Model file for the job. Use its own axes, mm. A direction names the side the tool comes from. Coordinates: 2 decimals unless noted, no trailing zeros. Order: outer loops, then holes, each group sorted by start corner. A loop starts at its lowest first (then second) coordinate and runs counter-clockwise, first axis right, second up. Notation, with made-up numbers: (88, 45) -> (115, 45) arc R24 cw to (115, 76) -> close; hole circle Ø5 at (17, 63.5). An arc over 180 degrees is marked (long way). Use CSV: the item, a comma, the result in double quotes. Start each with the question number.
(1) Cut at D-D on x = 20.5. Write the cut outline in (y, z), plus the area to 3 significant figures.
(2) Cut at B-B on x = 30.5. Write the cut outline in (y, z).
(3) Tool access for faces 4 (the flat face through (-12, -19, 3)), 5 (the cylindrical face through (-19.22, -24.79, 18.5)), 6 (the flat face through (-28, -20, 7.297)): list every direction of +Z, -Z, +X, -X, +Y, -Y with a clear straight run to the whole face (end or side of a thin tool).
(4) Probe L1, parallel to X at y = -21.5, z = 15; L2, parallel to X at y = -25.55, z = 17; L3, parallel to Y at x = 41, z = 17.25. List the from-to ranges inside material, lowest first.
(5) Cut at C-C on z = 10.25. Give the number of separate pieces and of enclosed holes in the cut face, plus the area to 3 significant figures.
(6) Pull direction Z, two halves, no side cores. Call faces 1 (the flat face through (-31, -16, 17)), 2 (the flat face through (-31, -28, 12)), 3 (the conical face through (40.656, 18.045, 6.007)): pulls with the +Z half, pulls with the -Z half, needs draft (parallel to the pull), parting line crosses it, or undercut.
(7) Pin check, flat tips, straight feed: pin 1 Ø4 at (x, z) = (15, 4) entering from -Y; pin 2 Ø1 at (x, y) = (12.5, -26) entering from +Z; pin 3 Ø3 at (x, z) = (-34.5, 14) entering from -Y; pin 4 Ø1.5 at (x, y) = (24.5, -17) entering from -Z. Stop position of each tip, or through.
(8) Cut at A-A on y = -20. Write the cut outline in (x, z), plus the area to 3 significant figures.
```python
from build123d import *

# Parameters (mm, degrees)
SKETCH1_W            = 92
SKETCH1_H            = 55
BODY_DEPTH           = 25
SKETCH2_R            = 9.75
BATTERY_DEPTH        = 37
SKETCH3_W            = 33
SKETCH3_H            = 8
CONTROLLER_DEPTH     = 22
CUT_EXTRUDE3_REACH   = 77.934
SKETCH4_R            = 4
CONNECTOR_REACH      = 77.934
SKETCH5_W            = 9
SKETCH5_H            = 10.5
SKETCH6_W            = 26
SKETCH6_H            = 6
CHARGER_DEPTH        = 22
CHGLED_REACH         = 77.934
SKETCH7_R            = 1.5
SKETCH8_W            = 20
SKETCH8_H            = 25
BOSS_EXTRUDE1_DEPTH  = 6
BOSS_EXTRUDE1_TAPER  = 30
SKETCH9_W            = 10
SKETCH9_H            = 14
CUT_EXTRUDE7_DEPTH   = 15
SKETCH10_W           = 8.515500197
SKETCH10_H           = 4.030526349
CUT_EXTRUDE8_DEPTH   = 15
SKETCH11_W           = 3
SKETCH11_H           = 48.5
CUT_EXTRUDE9_DEPTH   = 102.050729983
LPATTERN1_COUNT      = 2
LPATTERN1_PITCH      = 82
LPATTERN1_COUNT_DIR2 = 2
LPATTERN1_PITCH_DIR2 = 34
FILLET1_R            = 2
SKETCH14_R           = 2.730125357
CUT_EXTRUDE10_DEPTH  = 10


with BuildPart() as part:
    # Sketch1 → Body (new body)
    with BuildSketch(Plane.XY):
        Rectangle(SKETCH1_W, SKETCH1_H)
    extrude(amount=BODY_DEPTH)

    # Sketch2 → Battery (cut, symmetric)
    with BuildSketch(Plane(origin=(0, 0, 0), x_dir=(0, 0, -1), z_dir=(1, 0, 0))):
        with BuildLine():
            Line((-12, 3.5), (-12, 5))
            ThreePointArc((-12, 5), (-21.75, 14.75), (-12, 24.5))
            Line((-12, 24.5), (-28.22158826, 24.5))
            Line((-28.22158826, 24.5), (-28.22158826, -16))
            Line((-28.22158826, -16), (-12, -16))
            ThreePointArc((-12, -16), (-21.75, -6.25), (-12, 3.5))
        make_face()
        with Locations((-12, -6.25)):
            Circle(SKETCH2_R)
        with Locations((-12, 14.75)):
            Circle(SKETCH2_R)
    extrude(amount=BATTERY_DEPTH, both=True, mode=Mode.SUBTRACT)

    # Sketch3 → Controller (cut)
    with BuildSketch(Plane.XY.offset(25)):
        with Locations((20.5, -20)):
            Rectangle(SKETCH3_W, SKETCH3_H)
    extrude(amount=-CONTROLLER_DEPTH, mode=Mode.SUBTRACT)

    # Sketch4 → Cut-Extrude3 (cut, up to next)
    with BuildSketch(Plane.XZ.offset(27.5), mode=Mode.PRIVATE) as cut_extrude3_sk1:
        with Locations(Location((30.5, 12, 0), (0, 0, 270))):
            Circle(SKETCH4_R)
    cut_extrude3_tool1 = extrude(cut_extrude3_sk1.sketch, amount=-CUT_EXTRUDE3_REACH, mode=Mode.PRIVATE) & part.part
    add(cut_extrude3_tool1.solids().sort_by_distance((30.5, -27.5, 12))[0], mode=Mode.SUBTRACT)

    # Sketch5 → Connector (cut, up to next)
    with BuildSketch(Plane.XZ.offset(27.5), mode=Mode.PRIVATE) as connector_sk1:
        with Locations((13.5, 19.75)):
            Rectangle(SKETCH5_W, SKETCH5_H)
    connector_tool1 = extrude(connector_sk1.sketch, amount=-CONNECTOR_REACH, mode=Mode.PRIVATE) & part.part
    add(connector_tool1.solids().sort_by_distance((13.5, -27.5, 19.75))[0], mode=Mode.SUBTRACT)

    # Sketch6 → Charger (cut)
    with BuildSketch(Plane.XY.offset(25)):
        with Locations((-11.4, -19)):
            Rectangle(SKETCH6_W, SKETCH6_H)
    extrude(amount=-CHARGER_DEPTH, mode=Mode.SUBTRACT)

    # Sketch7 → ChgLED (cut, up to next)
    with BuildSketch(Plane(origin=(0, -27.5, 0), x_dir=(-1, 0, 0), z_dir=(0, -1, 0)), mode=Mode.PRIVATE) as chgled_sk1:
        with Locations(Location((19.286360004, -17, 0), (0, 0, 90))):
            Circle(SKETCH7_R)
    chgled_tool1 = extrude(chgled_sk1.sketch, amount=-CHGLED_REACH, mode=Mode.PRIVATE) & part.part
    add(chgled_tool1.solids().sort_by_distance((-19.28636, -27.5, 17))[0], mode=Mode.SUBTRACT)

    # Sketch8 → Boss-Extrude1 (add)
    with BuildSketch(Plane.XZ.offset(27.5)):
        with Locations((-36, 12.5)):
            Rectangle(SKETCH8_W, SKETCH8_H)
    extrude(amount=BOSS_EXTRUDE1_DEPTH, taper=BOSS_EXTRUDE1_TAPER)

    # Sketch9 → Cut-Extrude7 (cut)
    with BuildSketch(Plane.XZ.offset(33.5)):
        with Locations((-36, 12.5)):
            Rectangle(SKETCH9_W, SKETCH9_H)
    extrude(amount=-CUT_EXTRUDE7_DEPTH, mode=Mode.SUBTRACT)

    # Sketch10 → Cut-Extrude8 (cut)
    with BuildSketch(Plane(origin=(-24.4, 0, 0), x_dir=(0, 0, -1), z_dir=(1, 0, 0))):
        with Locations((-11.554387417, -19.984736826)):
            Rectangle(SKETCH10_W, SKETCH10_H)
    extrude(amount=-CUT_EXTRUDE8_DEPTH, mode=Mode.SUBTRACT)

    # Sketch11 → Cut-Extrude9 (cut, through all)
    with BuildSketch(Plane(origin=(46, 0, 0), x_dir=(0, 0, -1), z_dir=(1, 0, 0))):
        with Locations((-23.5, 0.25)):
            Rectangle(SKETCH11_W, SKETCH11_H)
    extrude(amount=-CUT_EXTRUDE9_DEPTH, mode=Mode.SUBTRACT)

    # Sketch13 → 4.0mm Dowel Hole1 (revolve, cut)
    with BuildSketch(Plane(origin=(41, 18, 22), x_dir=(0, -1, 0), z_dir=(1, 0, 0))):
        Polygon((0, 0), (0, 16.201721238), (2, 15), (2, 0), align=None)
    f_4_0mm_dowel_hole1 = revolve(axis=Axis((41, 18, 28.35), (0, 0, -1)), mode=Mode.SUBTRACT)

    # LPattern1: 4.0mm Dowel Hole1 2 × 2
    with Locations(*[(-i * LPATTERN1_PITCH, -j * LPATTERN1_PITCH_DIR2, 0) for i in range(LPATTERN1_COUNT) for j in range(LPATTERN1_COUNT_DIR2) if (i, j) != (0, 0)]):
        add(f_4_0mm_dowel_hole1, mode=Mode.SUBTRACT)

    # Fillet1
    fillet1_edges = [part.edges().sort_by_distance(p)[0] for p in [
        (20.5, -16, 12),
    ]]
    fillet(fillet1_edges, radius=FILLET1_R - 0.0004)  # a hair under: the kernel refuses the full size
    fillet1_2_edges = [part.edges().sort_by_distance(p)[0] for p in [
        (-11.4, -16, 12),
    ]]
    fillet(fillet1_2_edges, radius=FILLET1_R - 0.0004)  # a hair under: the kernel refuses the full size

    # Sketch14 → Cut-Extrude10 (cut)
    with BuildSketch(Plane(origin=(0, 0, 0), x_dir=(0, 0, -1), z_dir=(1, 0, 0))):
        with Locations((-15.777227018, -15.298336579)):
            Circle(SKETCH14_R)
    extrude(amount=CUT_EXTRUDE10_DEPTH, mode=Mode.SUBTRACT)


solid = part.part
```
Outcome:
1,outline,"(-27.5, 0) -> (27.5, 0) -> (27.5, 25) -> (24.5, 25) -> (24.5, 12) arc R9.75 cw to (5, 12) -> (3.5, 12) arc R9.75 cw to (-12.68, 4.67) arc R2 ccw to (-16, 3.17) -> (-16, 3) -> (-24, 3) -> (-24, 25) -> (-27.5, 25) -> close"
1,area,"367 mm2"
2,outline,"(-27.5, 0) -> (27.5, 0) -> (27.5, 25) -> (24.5, 25) -> (24.5, 12) arc R9.75 cw to (5, 12) -> (3.5, 12) arc R9.75 cw to (-12.68, 4.67) arc R2 ccw to (-16, 3.17) -> (-16, 3) -> (-24, 3) -> (-24, 8) -> (-27.5, 8) -> close; (-27.5, 16) -> (-24, 16) -> (-24, 25) -> (-27.5, 25) -> close"
3,face 4,"+Z"
3,face 5,"-Y"
3,face 6,"none"
4,L1,"-46 to -41, 1.6 to 4, 37 to 46"
4,L2,"-46 to -41, -31 to -20.79, -17.79 to 9, 18 to 46"
4,L3,"-27.5 to -18, -14 to 16, 20 to 27.5"
5,separate pieces,"2"
5,enclosed holes,"5"
5,area,"1,630 mm2"
6,face 1,"needs draft"
6,face 2,"undercut"
6,face 3,"pulls with the +Z half"
7,pin 1,"y = -27.5"
7,pin 2,"z = 14.5"
7,pin 3,"y = -17.97"
7,pin 4,"z = 0"
8,outline,"(-46, 0) -> (46, 0) -> (46, 22) -> (37, 22) -> (37, 3) -> (4, 3) -> (4, 22) -> (1.6, 22) -> (1.6, 3) -> (-24.4, 3) -> (-24.4, 7.3) -> (-31, 7.3) -> (-31, 5.5) -> (-41, 5.5) -> (-41, 19.5) -> (-31, 19.5) -> (-31, 15.81) -> (-24.4, 15.81) -> (-24.4, 22) -> (-46, 22) -> close"
8,area,"707 mm2"
